Here's how the part is built. I have some questions about the finished solid (model axes, mm). A direction names the side the tool comes from. Give positions to 0.01 mm unless a question says otherwise; leave off trailing zeros. Loops run counter-clockwise (first coordinate to the right, second up) from the corner with the lowest first, then second, coordinate; pieces in that order, holes last.
Q1. Will these pins go through, and if not, where does the flat tip stop? P1, Ø10, axis at y = 12.7, z = -171.45, coming from the -X side; P2, Ø3, axis at y = 15, z = -173.5, coming from the +X side.
Q2. For faces 5 (the face through (63, 13, 0)), 6 (the face through (9.658, 12.979, -177.794)), 7 (the face through (117.608, 18.054, -22.464)), which set-ups out of +Z, -Z, +X, -X, +Y, -Y let a thin tool reach every point of the face, with its end or its side?
Q3. If we section it at A-A (z = -171.45): Please give me the cut outline in (x, y).
Q4. If we section it at C-C (y = 12.7): Please give me the cut outline in (x, z).
Q5. I need wall thicknesses on line 1 (Y direction, x = 119, z = -171.45); line 2 (Y direction, x = 116.5, z = -19.05); line 3 (Z direction, x = 12, y = 17). Which ranges of each line are inside material? Lowest first, please.
Q6. We'd pull the mould along Y, two halves only. Please class faces 1 (the face through (9.658, 15.132, -24.916)), 2 (the face through (63, 13, -190.5)), 3 (the face through (107.95, 13, -171)), 4 (the face through (63, 25.4, -97)): +Y half, -Y half, draft (parallel to the pull), parting line (faces both ways), or undercut.
Q7. If we section it at B-B (x = 10.5): Please give me the cut outline in (y, z), plus the area to 3 significant figures.
Q8. If we section it at D-D (z = -19.05): Please give me the cut outline in (x, y).
from build123d import *

# Parameters (mm, degrees)
SKETCH1_W           = 127
SKETCH1_H           = 190.5
BOSS_EXTRUDE1_DEPTH = 25.4
SKETCH2_R           = 6.35
CUT_EXTRUDE1_DEPTH  = 19.05
SKETCH3_R           = 4.741125957
CUT_EXTRUDE2_DEPTH  = 19.05
CUT_EXTRUDE3_START  = -19.05
SKETCH8_R           = 6.35
CUT_EXTRUDE3_DEPTH  = 19.05


with BuildPart() as part:
    # Sketch1 → Boss-Extrude1 (new body)
    with BuildSketch(Plane(origin=(0, 0, 0), x_dir=(1, 0, 0), z_dir=(0, 1, 0))):
        with Locations((63.5, 95.25)):
            Rectangle(SKETCH1_W, SKETCH1_H)
    extrude(amount=BOSS_EXTRUDE1_DEPTH)

    # Sketch2 → Cut-Extrude1 (cut)
    with BuildSketch(Plane(origin=(127, 0, 0), x_dir=(0, 0, -1), z_dir=(1, 0, 0))):
        with Locations((19.05, 12.7)):
            Circle(SKETCH2_R)
    extrude(amount=-CUT_EXTRUDE1_DEPTH, mode=Mode.SUBTRACT)

    # Sketch3 → Cut-Extrude2 (cut)
    with BuildSketch(Plane(origin=(127, 0, 0), x_dir=(0, 0, -1), z_dir=(1, 0, 0))):
        with Locations((171.45, 12.7)):
            Circle(SKETCH3_R)
    extrude(amount=-CUT_EXTRUDE2_DEPTH, mode=Mode.SUBTRACT)

    # Sketch8 → Cut-Extrude3 (cut)
    with BuildSketch(Plane.ZY.offset(CUT_EXTRUDE3_START)):
        with Locations((-171.45, 12.7)):
            Circle(SKETCH8_R)
        with Locations(Location((-19.05, 12.7, 0), (0, 0, 180))):
            Circle(SKETCH8_R)
    extrude(amount=CUT_EXTRUDE3_DEPTH, mode=Mode.SUBTRACT)


solid = part.part
Check sheet entries:
1. P1: stops at x = 19.05
1. P2: stops at x = 107.95
2. face 5: +Z, +X, -X, +Y, -Y
2. face 6: -X
2. face 7: +X
3. outline: (0, 0) - (127, 0) - (127, 7.96) - (107.95, 7.96) - (107.95, 17.44) - (127, 17.44) - (127, 25.4) - (0, 25.4) - (0, 19.05) - (19.05, 19.05) - (19.05, 6.35) - (0, 6.35) - close
4. outline: (0, -190.5) - (127, -190.5) - (127, -176.19) - (107.95, -176.19) - (107.95, -166.71) - (127, -166.71) - (127, -25.4) - (107.95, -25.4) - (107.95, -12.7) - (127, -12.7) - (127, 0) - (0, 0) - (0, -12.7) - (19.05, -12.7) - (19.05, -25.4) - (0, -25.4) - (0, -165.1) - (19.05, -165.1) - (19.05, -177.8) - (0, -177.8) - close
5. line 1: y = 0 to 7.96, 17.44 to 25.4
5. line 2: y = 0 to 6.35, 19.05 to 25.4
5. line 3: z = -190.5 to -176.12, -166.78 to -23.72, -14.38 to 0
6. face 1: undercut
6. face 2: draft
6. face 3: undercut
6. face 4: +Y half
7. outline: (0, -190.5) - (25.4, -190.5) - (25.4, 0) - (0, 0) - close; hole circle Ø12.7 at (12.7, -171.45); hole circle Ø12.7 at (12.7, -19.05)
7. area: 4,590 mm2
8. outline: (0, 0) - (127, 0) - (127, 6.35) - (107.95, 6.35) - (107.95, 19.05) - (127, 19.05) - (127, 25.4) - (0, 25.4) - (0, 19.05) - (19.05, 19.05) - (19.05, 6.35) - (0, 6.35) - close
